Geometry check sheet. Reference: the model listing, model coordinates, mm. Coordinates: 2 decimals unless noted, no trailing zeros. Write each loop counter-clockwise with the first axis right and the second up, starting at its lowest first coordinate (ties: lowest second). Pieces come first, ordered by that corner, then holes. Notation, with made-up numbers: M -32,44.25 L -1,44.25 A4 cw -1,50.25 Z; hole C -18.75,41 d11. An arc over 180 degrees is marked long. Put each result on its own line as item: value. Start each with the question number.
1) Gauge pin test, flat ends, axial feed: pin 1 (1.8 mm diameter, centred on y = 2, z = 3, fed in from -X); pin 2 (3 mm diameter, centred on y = 1.5, z = 3, fed in from +X); pin 3 (1.5 mm diameter, centred on x = -44.5, z = 3.5, fed in from -Y). Record the tip position at first contact, or that the pin passes through.
2) Scan lines: line 1 along X through (y, z) = (34, 3.9); line 2 along Y through (x, z) = (-196, 4.45). Record each from-to range of solid material in increasing order.
3) Cross-section at A-A on y = 37. Record the cut outline in (x, z).
4) Cross-section at B-B on x = -5. Record the cut outline in (y, z).
from build123d import *

# Parameters (mm, degrees)
BOSS_EXTRUDE1_DEPTH = 6
SKETCH3_W           = 6
SKETCH3_H           = 20
BOSS_EXTRUDE2_DEPTH = 6


with BuildPart() as part:
    # Sketch1 → Boss-Extrude1 (new body)
    with BuildSketch(Plane.XY):
        Polygon((-225, 0), (-204, 0), (-204, 6), (-180, 6), (-180, 0), (-156, 0), (-156, 6), (-132, 6), (-132, 0), (-108, 0), (-108, 6), (-84, 6), (-84, 0), (-60, 0), (-60, 6), (-36, 6), (-36, 0), (-12, 0), (-12, 6), (12, 6), (12, 0), (36, 0), (36, 6), (60, 6), (60, 0), (84, 0), (84, 6), (108, 6), (108, 0), (132, 0), (132, 6), (156, 6), (156, 0), (180, 0), (180, 6), (204, 6), (204, 0), (225, 0), (225, 72), (204, 72), (204, 66), (180, 66), (180, 72), (156, 72), (156, 66), (132, 66), (132, 72), (108, 72), (108, 66), (84, 66), (84, 72), (60, 72), (60, 66), (36, 66), (36, 72), (12, 72), (12, 66), (-12, 66), (-12, 72), (-36, 72), (-36, 66), (-60, 66), (-60, 72), (-84, 72), (-84, 66), (-108, 66), (-108, 72), (-132, 72), (-132, 66), (-156, 66), (-156, 72), (-180, 72), (-180, 66), (-204, 66), (-204, 72), (-225, 72), align=None)
    extrude(amount=BOSS_EXTRUDE1_DEPTH)

    # Sketch3 → Boss-Extrude2 (add)
    with BuildSketch(Plane.XY.offset(6)):
        with Locations((-228, 16)):
            Rectangle(SKETCH3_W, SKETCH3_H)
        with Locations((-228, 56)):
            Rectangle(SKETCH3_W, SKETCH3_H)
        with Locations((228, 16)):
            Rectangle(SKETCH3_W, SKETCH3_H)
        with Locations((228, 56)):
            Rectangle(SKETCH3_W, SKETCH3_H)
    extrude(amount=-BOSS_EXTRUDE2_DEPTH)


solid = part.part
Answer key:
1. pin 1: stops at x = -225
1. pin 2: stops at x = 225
1. pin 3: stops at y = 6
2. line 1: x = -225 to 225
2. line 2: y = 6 to 66
3. outline: M -225,0 L 225,0 L 225,6 L -225,6 Z
4. outline: M 6,0 L 66,0 L 66,6 L 6,6 Z
